from build123d import *

# Parameters (mm, degrees)
F0_R     = 29.25
F1_DEPTH = 5
F3_DEPTH = 41
F6_DEPTH = 25.4


with BuildPart() as f1:
    # F0 (on Top) → F1 (new body)
    with BuildSketch(Plane.XY):
        Circle(F0_R)
    extrude(amount=F1_DEPTH)

    # F2 (on face) → F3 (join)
    with BuildSketch(Plane.XY.offset(5)):
        with BuildLine():
            Line((18.559394, 5.10993), (4.006055, 18.828543))
            ThreePointArc((4.006055, 18.828543), (-13.204164, -14.007589), (18.559394, 5.10993))
        make_face()
        with BuildLine():
            ThreePointArc((14.467536, 3.961112), (-10.288959, -10.915004), (3.10065, 14.676034))
            Line((3.10065, 14.676034), (14.467536, 3.961112))
        make_face(mode=Mode.SUBTRACT)
    extrude(amount=F3_DEPTH)

    # F5 (on face) → F6 (cut)
    with BuildSketch(Plane(origin=(0, 0, 0), x_dir=(1, 0, 0), z_dir=(0, 0, -1))):
        with BuildLine():
            Line((1.419319, -6.319578), (6.224832, -1.789692))
            ThreePointArc((6.224832, -1.789692), (-4.442773, 4.713099), (1.419319, -6.319578))
        make_face()
    extrude(amount=-F6_DEPTH, mode=Mode.SUBTRACT)


solid = f1.part
Read the model definition and answer for the solid it produces. Units are mm, in the model's axes. A direction names the side the tool comes from. Give positions to 0.01 mm unless a question says otherwise; leave off trailing zeros. Write each loop counter-clockwise with the first axis right and the second up, starting at its lowest first coordinate (ties: lowest second). Pieces come first, ordered by that corner, then holes. Notation, with made-up numbers: M 22.5,28.25 L 59.5,28.25 A30 cw 59.5,63.25 Z; hole C 31.5,64 d5. An arc over 180 degrees is marked long. One line per item, written item: value. Start each with the question number.
(1) Determine the mould class of faces 1 (the flat face through (0, 7, 0)), 2 (the cylindrical face through (-9.89, -11.28, 25.21)), 3 (the cylindrical face through (-6.341, -28.554, 2.465)) for opening direction Y: pulls with the +Y half, pulls with the -Y half, needs draft (parallel to the pull), parting line crosses it, or undercut.
(2) Find section C-C (x = -7.5). Determine the outline of the cut face in (y, z).
(3) Flat-ended cylindrical pins translate along their axes: pin 1 Ø1.5 at (y, z) = (11.5, 7.5) entering from +X; pin 2 Ø2 at (x, y) = (7, -19) entering from -Z; pin 3 Ø6 at (x, z) = (-19, 33.5) entering from -Y; pin 4 Ø2 at (y, z) = (14.5, 21) entering from -X. Find the tip coordinate at first contact, or state that the pin passes through.
(4) Find section D-D (z = 22.5). Determine the outline of the cut face in (x, y).
(5) Find section A-A (x = 0). Determine the outline of the cut face in (y, z).
(6) Find the intervals of material crossed by line 1 (X direction, y = 0, z = 37); line 2 (Y direction, x = 0, z = 3), in increasing order.
(7) A tool of negligible diameter and unlimited length cuts with its end or side. For faces 4 (the flat face through (13, 13, 5)), 5 (the flat face through (3.788, 4.086, 2.465)), 6 (the flat face through (11.385, 11.873, 25.213)), from which of +Z, -Z, +X, -X, +Y, -Y can it reach the whole face along a straight path? Write none if from no direction.
Results below:
1. face 1: needs draft
1. face 2: undercut
1. face 3: parting line crosses it
2. outline: M -28.27,0 L 28.27,0 L 28.27,5 L 17.73,5 L 17.73,46 L 12.99,46 L 12.99,5 L -12.99,5 L -12.99,46 L -17.73,46 L -17.73,5 L -28.27,5 Z
3. pin 1: stops at x = 12.58
3. pin 2: stops at z = 0
3. pin 3: stops at y = -10.7
3. pin 4: stops at x = -13.72
4. outline: M 4.01,18.83 A19.25 ccw long 18.56,5.11 Z; hole M 3.1,14.68 A15 ccw long 14.47,3.96 Z
5. outline: M -29.25,0 L -6.48,0 L -6.48,5 L -15,5 L -15,46 L -19.25,46 L -19.25,5 L -29.25,5 Z; M 6.48,0 L 29.25,0 L 29.25,5 L 19.25,5 L 19.25,46 L 15,46 L 15,5 L 6.48,5 Z
6. line 1: x = -19.25 to -15, 15 to 19.25
6. line 2: y = -29.25 to -6.48, 6.48 to 29.25
7. face 4: +Z
7. face 5: +Z, -Z
7. face 6: +Z, +X, +Y
